Solid Edge part; units mm, degrees
sketch "Sketch1" plane through (0, 0, 0) normal (0, 0, 1) x (1, 0, 0)
  line L0 (4.7625, -4.7625) -> (4.7625, 4.7625)
  line L1 (4.7625, 4.7625) -> (-4.7625, 4.7625)
  line L2 (-4.7625, 4.7625) -> (-4.7625, -4.7625)
  line L3 (-4.7625, -4.7625) -> (4.7625, -4.7625)
extrude "Protrusion1" add sketch "Sketch1" along normal blind 9.525
sketch "Sketch2" plane through (0, 0, 0) normal (0, 0, -1) x (1, 0, 0)
  circle A0 centre (0, 0) radius 3.429
extrude "ExtrudedCutout_1" cut sketch "Sketch2" against normal blind 6.35
sketch "Sketch3" plane through (4.7625, 0, 4.7625) normal (1, 0, 0) x (0, 1, 0)
  line L0 (-1.27, 0.3175) -> (-1.27, -4.7625)
  line L1 (-1.27, -4.7625) -> (0, -4.7625)
  line L2 (0, -4.7625) -> (1.27, -4.7625)
  line L3 (1.27, -4.7625) -> (1.27, 0.3175)
  line L4 (1.27, 0.3175) -> (-1.27, 0.3175)
extrude "ExtrudedProtrusion_3" add sketch "Sketch3" along normal blind 4.445
sketch "Sketch4" plane through (6.985, -1.27, 2.54) normal (0, -1, 0) x (1, 0, 0)
  circle A0 centre (0, 0) radius 1.5875
extrude "Cutout1" cut sketch "Sketch4" against normal up to vertex (2.54 mm away)
mirror "Mirror1" about plane through (0, 0, 0) normal (1, 0, 0) of "ExtrudedProtrusion_3", "Cutout1"
fillet "Round_1" radius 0.635 14 edges at (4.7625, -4.7625, 4.7625) (4.7625, 4.7625, 4.7625) (-4.7625, -4.7625, 4.7625) (-4.7625, 4.7625, 4.7625) (9.2075, 1.27, 2.54) (9.2075, -1.27, 2.54) (-9.2075, 1.27, 2.54) (-9.2075, -1.27, 2.54) (4.7625, 0, 5.08) (-4.7625, 0, 5.08) (4.7625, 0, 9.525) (0, 4.7625, 9.525) (-4.7625, 0, 9.525) (0, -4.7625, 9.525)
properties material "ABS Plastic, medium impact"
Here's how the part is built. I have some questions about the finished solid (model axes, mm). A direction names the side the tool comes from. Coordinates: 2 decimals unless noted, no trailing zeros. Order: outer loops, then holes, each group sorted by start corner. A loop starts at its lowest first (then second) coordinate and runs counter-clockwise, first axis right, second up.
1) I need wall thicknesses on line 1 (X direction, y = 0.25, z = 3.5); line 2 (Z direction, x = -7, y = 0.5); line 3 (X direction, y = 0, z = 4.5). Which ranges of each line are inside material? Lowest first, please.
2) We'd pull the mould along X, two halves only. Please class faces 1 (the face through (-4.762, 0, 6)), 2 (the face through (9.208, 0, 3)), 3 (the face through (0, 0, 6.35)): +X half, -X half, draft (parallel to the pull), parting line (faces both ways), or undercut.
3) Imagine slicing it at B-B on z = 4.75. List the corners of the cut face in (x, y) for me, and give its area (3 significant figures).
4) Which directions (+Z, -Z, +X, -X, +Y, -Y) give clear straight access to the entire face, cutting with the end or side of a thin tool? Please do faces 4 (the face through (5, 1.27, 2)), 5 (the face through (-7, 0, 5.08)), 6 (the face through (5, -1.27, 3)), 7 (the face through (-0.74, 3.35, 3.13)).
5) Will these pins go through, and if not, where does the flat tip stop? pin 1 (1.3 mm diameter, centred on x = 8, y = -0.5, fed in from +Z); pin 2 (4 mm diameter, centred on x = 5.5, y = -1.5, fed in from -Z); pin 3 (2 mm diameter, centred on x = -6.5, z = 3.5, fed in from +Y); pin 4 (4 mm diameter, centred on x = 7.5, z = 2, fed in from -Y).
6) Imagine slicing it at D-D on x = 6.25. List the corners of the cut face in (y, z) for me.
7) Imagine slicing it at A-A on z = 2.54. State how many separate pieces and enclosed holes the cut face has, and give its area (3 significant figures).
Response values:
1. line 1: x = -9.21 to -8.25, -5.72 to -3.42, 3.42 to 5.72, 8.25 to 9.21
1. line 2: z = 0 to 0.95, 4.13 to 5.08
1. line 3: x = -9.21 to -3.43, 3.43 to 9.21
2. face 1: -X half
2. face 2: +X half
2. face 3: undercut
3. outline: (-9.21, -0.64) arc R0.63 ccw to (-8.57, -1.27) - (-4.76, -1.27) - (-4.76, -4.13) arc R0.63 ccw to (-4.13, -4.76) - (4.13, -4.76) arc R0.63 ccw to (4.76, -4.13) - (4.76, -1.27) - (8.57, -1.27) arc R0.63 ccw to (9.21, -0.64) - (9.21, 0.64) arc R0.63 ccw to (8.57, 1.27) - (4.76, 1.27) - (4.76, 4.13) arc R0.63 ccw to (4.13, 4.76) - (-4.13, 4.76) arc R0.63 ccw to (-4.76, 4.13) - (-4.76, 1.27) - (-8.57, 1.27) arc R0.63 ccw to (-9.21, 0.64) - close; hole circle Ø6.86 at (0, 0)
3. area: 75.7 mm2
4. face 4: +Z, -Z, +X, +Y
4. face 5: +Z, -X, +Y, -Y
4. face 6: +Z, -Z, +X, -Y
4. face 7: -Z
5. pin 1: stops at z = 5.08
5. pin 2: stops at z = 0
5. pin 3: stops at y = 1.27
5. pin 4: stops at y = -1.27
6. outline: (-1.27, 0) - (1.27, 0) - (1.27, 1.13) - (-1.27, 1.13) - close; (-1.27, 3.95) - (1.27, 3.95) - (1.27, 5.08) - (-1.27, 5.08) - close
7. separate pieces: 3
7. enclosed holes: 1
7. area: 59.5 mm2
